Verification items for this drawing (mm, ordinates from the low corner). A direction names the side the tool comes from. Coordinates: 2 decimals unless noted, no trailing zeros. Write each loop counter-clockwise with the first axis right and the second up, starting at its lowest first coordinate (ties: lowest second). Pieces come first, ordered by that corner, then holes. Notation, with made-up numbers: (25.5, -23) -> (30.5, -23) arc R29 ccw to (30.5, 2) -> close; hole circle Ø3 at (-15.75, 44). An arc over 180 degrees is marked (long way). Answer as CSV lines item,"result".
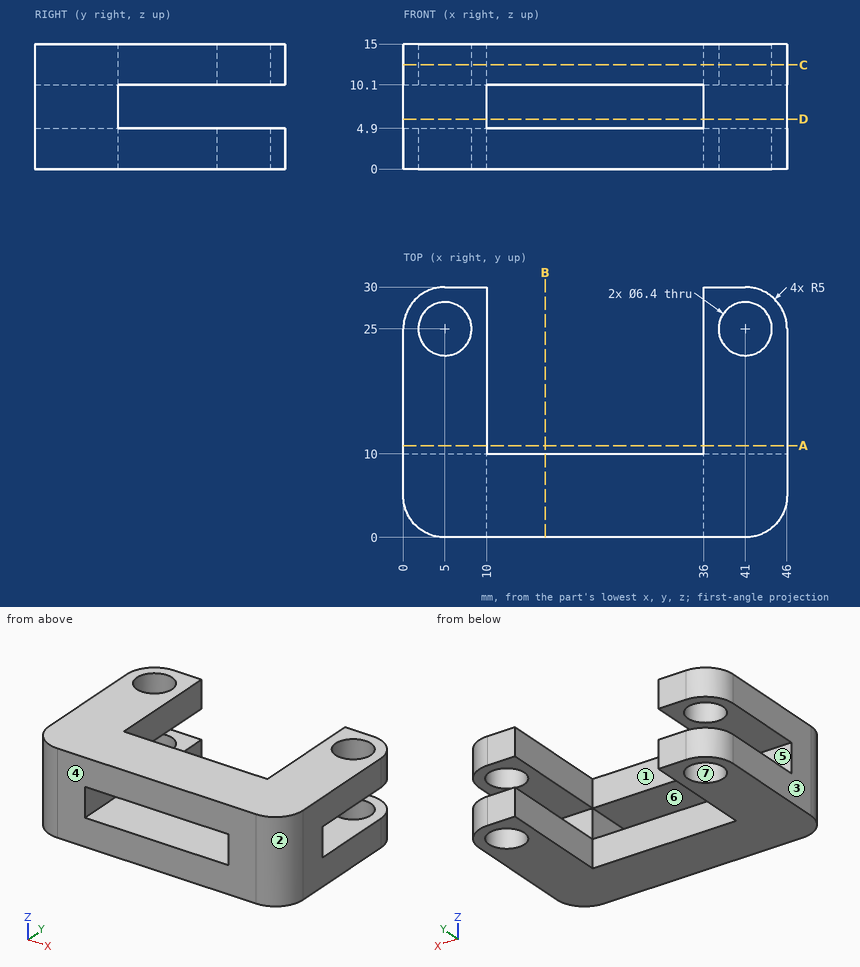
Item 1: Cross-section at C-C, the plane z = 12.5. Record the cut outline in (x, y).
Responses:
outline,"(0, 5) arc R5 ccw to (5, 0) -> (41, 0) arc R5 ccw to (46, 5) -> (46, 25) arc R5 ccw to (41, 30) -> (36, 30) -> (36, 10) -> (10, 10) -> (10, 30) -> (5, 30) arc R5 ccw to (0, 25) -> close; hole circle Ø6.4 at (5, 25); hole circle Ø6.4 at (41, 25)"
Item 2: Cross-section at B-B, the plane x = 17. Record the cut outline in (y, z), plus the area to 3 significant figures.
Responses:
outline,"(0, 0) -> (10, 0) -> (10, 4.9) -> (0, 4.9) -> close; (0, 10.1) -> (10, 10.1) -> (10, 15) -> (0, 15) -> close"
area,"98.0 mm2"
Item 3: Set-up check for the marked faces 5, 6 and 7: record each of +Z, -Z, +X, -X, +Y, -Y from which the full face is reachable in a straight line by a thin tool's end or side.
Responses:
face 5,"+X, -X, +Y"
face 6,"+Y, -Y"
face 7,"+Z, -Z"
Item 4: Depth check by flat-ended pin: pin 1 Ø2 at (x, z) = (14, 11) entering from +Y; pin 2 Ø5 at (x, y) = (41, 25) entering from +Z; pin 3 Ø1.6 at (y, z) = (3.5, 8.5) entering from +X. Enter the tip coordinate at first touch or a pass-through.
Responses:
pin 1,"stops at y = 10"
pin 2,"passes through"
pin 3,"stops at x = 45.95"
Item 5: Cross-section at D-D, the plane z = 6. Record the cut outline in (x, y).
Responses:
outline,"(0, 5) arc R5 ccw to (5, 0) -> (10, 0) -> (10, 10) -> (0, 10) -> close; (36, 0) -> (41, 0) arc R5 ccw to (46, 5) -> (46, 10) -> (36, 10) -> close"
Item 6: Release check for a two-part mould opening along X. For the marked faces 1, 2, 3 and 4 record: +X half, -X half, draft (parallel to the pull), parting line (faces both ways), or undercut.
Responses:
face 1,"undercut"
face 2,"+X half"
face 3,"-X half"
face 4,"draft"
Item 7: Thickness scan on probe 1 along Z at (x, y) = (20, 5); probe 2 along Y at (x, z) = (34.5, 2.5); probe 3 along X at (y, z) = (16, 12.5). Record the ranges inside material, lowest first.
Responses:
probe 1,"z = 0 to 4.9, 10.1 to 15"
probe 2,"y = 0 to 10"
probe 3,"x = 0 to 10, 36 to 46"
Item 8: Cross-section at A-A, the plane y = 11. Record the cut outline in (x, z), plus the area to 3 significant figures.
Responses:
outline,"(0, 0) -> (10, 0) -> (10, 4.9) -> (0, 4.9) -> close; (0, 10.1) -> (10, 10.1) -> (10, 15) -> (0, 15) -> close; (36, 0) -> (46, 0) -> (46, 4.9) -> (36, 4.9) -> close; (36, 10.1) -> (46, 10.1) -> (46, 15) -> (36, 15) -> close"
area,"196 mm2"
